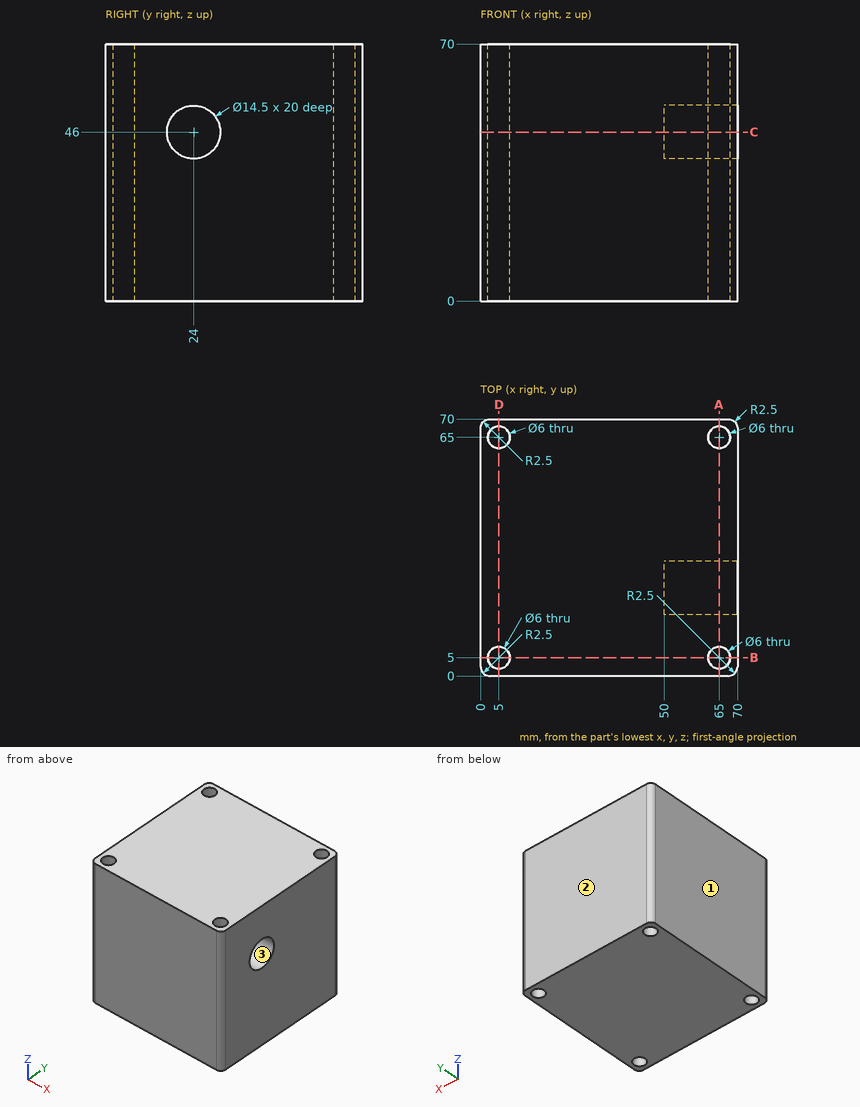
Study the drawing (mm; zero at the part's minimum x, y, z) and answer. Round coordinates to 2 decimals unless told otherwise and drop trailing zeros. Loops run counter-clockwise (first coordinate to the right, second up) from the corner with the lowest first, then second, coordinate; pieces in that order, holes last. Notation, with made-up numbers: (35.25, -23.75) -> (77.25, -23.75) arc R25 ccw to (77.25, 12.25) -> close; hole circle Ø5 at (-1.75, 19.5). An arc over 180 degrees is marked (long way). Use one line per item in the form item = value.
1. The part is cut by section C-C on z = 46. Determine the outline of the cut face in (x, y), and give its area (3 significant figures).
Answer key:
outline = (0, 2.5) arc R2.5 ccw to (2.5, 0) -> (67.5, 0) arc R2.5 ccw to (70, 2.5) -> (70, 16.75) -> (50, 16.75) -> (50, 31.25) -> (70, 31.25) -> (70, 67.5) arc R2.5 ccw to (67.5, 70) -> (2.5, 70) arc R2.5 ccw to (0, 67.5) -> close; hole circle Ø6 at (5, 5); hole circle Ø6 at (5, 65); hole circle Ø6 at (65, 5); hole circle Ø6 at (65, 65)
area = 4,490 mm²
2. A flat-ended cylindrical pin translates along its axis: pin 1 Ø23 at (y, z) = (24, 46) entering from +X. Find the tip coordinate at first contact, or state that the pin passes through.
Answer key:
pin_1 = 70
3. Find the intervals of material crossed by probe 1 along Y at (x, z) = (65, 26); probe 2 along Y at (x, z) = (65, 44), in increasing order. Write a range as [from, to].
Answer key:
probe_1 = [0, 2], [8, 62], [68, 70]
probe_2 = [0, 2], [8, 17.03], [30.97, 62], [68, 70]
4. For a pull along Y with two mould halves and no side action, classify the marked faces 1, 2 and 3 as released by +Y, released by -Y, zero draft, split by the parting line, or undercut.
Answer key:
face_1 = zero draft
face_2 = released by +Y
face_3 = undercut
5. The part is cut by section B-B on y = 5. Determine the outline of the cut face in (x, z), and give its area (3 significant figures).
Answer key:
outline = (0, 0) -> (2, 0) -> (2, 70) -> (0, 70) -> close; (8, 0) -> (62, 0) -> (62, 70) -> (8, 70) -> close; (68, 0) -> (70, 0) -> (70, 70) -> (68, 70) -> close
area = 4,060 mm²
6. The part is cut by section A-A on x = 65. Determine the outline of the cut face in (y, z).
Answer key:
outline = (0, 0) -> (2, 0) -> (2, 70) -> (0, 70) -> close; (8, 0) -> (62, 0) -> (62, 70) -> (8, 70) -> close; (68, 0) -> (70, 0) -> (70, 70) -> (68, 70) -> close; hole circle Ø14.5 at (24, 46)
